```python
from build123d import *

# Parameters (mm, degrees)
SKETCH1_W           = 92.0496
SKETCH1_H           = 32.2834
BOSS_EXTRUDE1_DEPTH = 4.7625
SKETCH2_R           = 1.1303
CUT_EXTRUDE1_DEPTH  = 19.05
SKETCH3_R           = 1.1303
CUT_EXTRUDE2_DEPTH  = 94.57544948


with BuildPart() as part:
    # Sketch1 → Boss-Extrude1 (new body)
    with BuildSketch(Plane.XY):
        Rectangle(SKETCH1_W, SKETCH1_H)
    extrude(amount=BOSS_EXTRUDE1_DEPTH)

    # Sketch2 → Cut-Extrude1 (cut)
    with BuildSketch(Plane.XZ.offset(16.1417)):
        with Locations(Location((-20.6248, 2.38125, 0), (0, 0, 270))):
            Circle(SKETCH2_R)
        with Locations(Location((20.6248, 2.38125, 0), (0, 0, 270))):
            Circle(SKETCH2_R)
    extrude(amount=-CUT_EXTRUDE1_DEPTH, mode=Mode.SUBTRACT)

    # Sketch3 → Cut-Extrude2 (cut, through all)
    with BuildSketch(Plane.ZY.offset(46.0248)):
        with Locations((2.38125, 7.5311)):
            Circle(SKETCH3_R)
        with Locations((2.38125, -5.8801)):
            Circle(SKETCH3_R)
    extrude(amount=-CUT_EXTRUDE2_DEPTH, mode=Mode.SUBTRACT)


solid = part.part
```
Design review of the part built by this model. Coordinates are the model's own, in mm. A direction names the side the tool comes from. Round coordinates to 2 decimals unless told otherwise and drop trailing zeros. Write each loop counter-clockwise with the first axis right and the second up, starting at its lowest first coordinate (ties: lowest second). Pieces come first, ordered by that corner, then holes.
Item 1: For faces 4 (the flat face through (-1, 0, 0)), 5 (the cylindrical face through (20.96, -11.08, 1.3)), list the 3-axis set-ups (+Z, -Z, +X, -X, +Y, -Y) from which the entire face can be reached by the end or side of a thin tool; tool diameter is ignored.
Item 2: We need section B-B on x = -2. Write out the cut boundary in (y, z), and give its area (3 significant figures).
Item 3: We need section A-A on y = 0. Write out the cut boundary in (x, z), and give its area (3 significant figures).
Item 4: The part is to be moulded in two halves that separate along X. For faces 1 (the flat face through (-46.025, 0, 2)), 2 (the cylindrical face through (21.745, -1.547, 2.528)), 3 (the cylindrical face through (-0.644, 7.098, 3.425)), say which applies: +X half, -X half, draft (parallel to the pull), parting line (faces both ways), or undercut.
Item 5: For probe 1 along X at (y, z) = (-13.5, 3); probe 2 along Y at (x, z) = (7, 3.15); probe 3 along Y at (x, z) = (4, 3.4), list the stretches that pass through material, from the lowest coordinate up.
Returned:
1. face 4: -Z, +X, -X, +Y, -Y
1. face 5: -Y
2. outline: (-16.14, 0) - (16.14, 0) - (16.14, 4.76) - (-16.14, 4.76) - close; hole circle Ø2.26 at (-5.88, 2.38); hole circle Ø2.26 at (7.53, 2.38)
2. area: 146 mm2
3. outline: (-46.02, 0) - (46.02, 0) - (46.02, 4.76) - (-46.02, 4.76) - close; hole circle Ø2.26 at (-20.62, 2.38); hole circle Ø2.26 at (20.62, 2.38)
3. area: 430 mm2
4. face 1: -X half
4. face 2: undercut
4. face 3: draft
5. probe 1: x = -46.02 to -21.57, -19.68 to 19.68, 21.57 to 46.02
5. probe 2: y = -16.14 to -6.71, -5.05 to 6.7, 8.36 to 16.14
5. probe 3: y = -16.14 to -6.37, -5.39 to 7.04, 8.02 to 16.14
